Geometry: final body of the model. Coordinates: model frame, mm. A direction names the side the tool comes from. Give positions to 0.01 mm unless a question says otherwise; leave off trailing zeros. Loops run counter-clockwise (first coordinate to the right, second up) from the corner with the lowest first, then second, coordinate; pieces in that order, holes last.
1. Material intervals for line 1 along Z through (x, y) = (0, -12.5); line 2 along X through (y, z) = (89, 9); line 3 along Y through (x, z) = (5, 0.5), sorted ascending.
2. Access query for faces 5 (the face through (0, -2, -3.9)), 6 (the face through (-10, -2, 7)), 7 (the face through (6.993, 119.404, -2.685)). Directions: +Z, -Z, +X, -X, +Y, -Y. A direction counts if a zero-diameter tool reaches every point of the face in a straight line with its end or side. Return the directions, or none.
3. Draft query along Z for faces 1 (the face through (-3.9, -2, 0)), 2 (the face through (6.993, -120.596, -2.685)), 3 (the face through (10, -2, 7)), 4 (the face through (0, -2, 3.9)). Return one class per face: +Z half, -Z half, draft (parallel to the pull), parting line (faces both ways), or undercut.
4. First-contact query: P1, Ø3, axis at x = -1.5, y = -16.5, coming from the -Z side; P2, Ø3, axis at y = -24, z = 0.5, coming from the -X side; P3, Ø6, axis at x = 0.5, y = -30, coming from the +Z side. Flat tips, straight axial feed; report the tip coordinate or a pass-through.
5. Section A-A, the plane z = 0. Output: boundary loops of the cut face in (x, y), then the cut area to 3 significant figures.
from build123d import *

# Parameters (mm, degrees)
F0_R     = 2.1
F1_DEPTH = 125
F2_R     = 2.75
F3_DEPTH = 6.1


with BuildPart() as f1:
    # F0 (on Front) → F1 (new body, symmetric)
    with BuildSketch(Plane.XZ):
        Polygon((3.9, 2.83934), (3.9, 3.9), (2.83934, 3.9), (-2.83934, 3.9), (-3.9, 3.9), (-3.9, 2.83934), (-3.9, -2.83934), (-3.9, -3.9), (-2.83934, -3.9), (2.83934, -3.9), (3.9, -3.9), (3.9, -2.83934), align=None)
        Circle(F0_R, mode=Mode.SUBTRACT)
        Polygon((2.83934, 3.9), (3.9, 3.9), (3.9, 2.83934), (6.56066, 5.5), (9.1, 5.5), (9.1, 3.125), (10, 4.58), (10, 10), (4.58, 10), (3.125, 9.1), (5.5, 9.1), (5.5, 6.56066), align=None)
        Polygon((-3.9, 3.9), (-2.83934, 3.9), (-5.5, 6.56066), (-5.5, 9.1), (-3.125, 9.1), (-4.58, 10), (-10, 10), (-10, 4.58), (-9.1, 3.125), (-9.1, 5.5), (-6.56066, 5.5), (-3.9, 2.83934), align=None)
        Polygon((6.56066, -5.5), (3.9, -2.83934), (3.9, -3.9), (2.83934, -3.9), (5.5, -6.56066), (5.5, -9.1), (3.125, -9.1), (4.58, -10), (10, -10), (10, -4.58), (9.1, -3.125), (9.1, -5.5), align=None)
        Polygon((-3.9, -3.9), (-3.9, -2.83934), (-6.56066, -5.5), (-9.1, -5.5), (-9.1, -3.125), (-10, -4.58), (-10, -10), (-4.58, -10), (-3.125, -9.1), (-5.5, -9.1), (-5.5, -6.56066), (-2.83934, -3.9), align=None)
    extrude(amount=F1_DEPTH, both=True)

    # F2 (on face) → F3 (join, through all)
    with BuildSketch(Plane.YZ.offset(10)):
        with Locations((-120, 0)):
            Circle(F2_R)
        with Locations((120, 0)):
            Circle(F2_R)
    extrude(amount=-F3_DEPTH)


solid = f1.part
Answers below:
1. line 1: z = -3.9 to -2.1, 2.1 to 3.9
1. line 2: x = -10 to -5.5, 5.5 to 10
1. line 3: y = -122.7 to -117.3, 117.3 to 122.7
2. face 5: -Z, +Y, -Y
2. face 6: +Z, -Z, -X, +Y, -Y
2. face 7: +X
3. face 1: undercut
3. face 2: undercut
3. face 3: draft
3. face 4: +Z half
4. P1: stops at z = -4.06
4. P2: stops at x = -3.9
4. P3: stops at z = 9.33
5. outline: (-3.9, -125) - (-2.1, -125) - (-2.1, 125) - (-3.9, 125) - close; (2.1, -125) - (3.9, -125) - (3.9, -122.75) - (10, -122.75) - (10, -117.25) - (3.9, -117.25) - (3.9, 117.25) - (10, 117.25) - (10, 122.75) - (3.9, 122.75) - (3.9, 125) - (2.1, 125) - close
5. area: 967 mm2
